Check sheet for the modelled part. Datum: model origin and axes. Units: mm. A direction names the side the tool comes from. Round coordinates to 2 decimals unless told otherwise and drop trailing zeros. Write each loop counter-clockwise with the first axis right and the second up, starting at its lowest first coordinate (ties: lowest second). Pieces come first, ordered by that corner, then holes. Notation, with made-up numbers: M 45.25,24.25 L 85.25,24.25 A22 cw 85.25,32.25 Z; hole C -24,4 d6. An arc over 180 degrees is marked long. One line per item, written item: value.
from build123d import *

# Parameters (mm, degrees)
F0_R     = 37
F0_R_2   = 35.5
F1_DEPTH = 1.5
F0_R_3   = 1.5
F2_DEPTH = 4


with BuildPart() as f1:
    # F0 (on Right) → F1 (new body, symmetric)
    with BuildSketch(Plane.YZ):
        Circle(F0_R)
        Circle(F0_R_2, mode=Mode.SUBTRACT)
    extrude(amount=F1_DEPTH, both=True)

    # F0 (on Right) → F2 (join, symmetric)
    with BuildSketch(Plane.YZ):
        Circle(F0_R_2)
        Circle(F0_R_3, mode=Mode.SUBTRACT)
    extrude(amount=F2_DEPTH, both=True)


solid = f1.part
Q1. Sectioned sample at D-D on z = 20. Enter the section's corners in (x, y).
Completed:
outline: M -4,-29.33 L -1.5,-29.33 L -1.5,-31.13 L 1.5,-31.13 L 1.5,-29.33 L 4,-29.33 L 4,29.33 L 1.5,29.33 L 1.5,31.13 L -1.5,31.13 L -1.5,29.33 L -4,29.33 Z
Q2. Sectioned sample at C-C on x = 3. Enter the section's corners in (y, z).
Completed:
outline: C 0,0 d71; hole C 0,0 d3
Q3. Sectioned sample at A-A on y = 0. Enter the section's corners in (x, z), and give its area (3 significant figures).
Completed:
outline: M -4,-35.5 L -1.5,-35.5 L -1.5,-37 L 1.5,-37 L 1.5,-35.5 L 4,-35.5 L 4,-1.5 L -4,-1.5 Z; M -4,1.5 L 4,1.5 L 4,35.5 L 1.5,35.5 L 1.5,37 L -1.5,37 L -1.5,35.5 L -4,35.5 Z
area: 553 mm^2
Q4. Depth check by flat-ended pin: P1, Ø1.8, axis at y = 0, z = 0, coming from the +X side; P2, Ø1, axis at x = 2.5, z = -26, coming from the -Y side; P3, Ø1.5, axis at x = 3, y = 14, coming from the -Z side; P4, Ø4, axis at x = 0, z = 7, coming from the -Y side. Enter the tip coordinate at first touch or a pass-through.
Completed:
P1: through
P2: y = -24.7
P3: z = -32.93
P4: y = -36.66
Q5. Scan lines: line 1 (Z direction, x = -1.25, y = 0); line 2 (Z direction, x = -2, y = -24); line 3 (Y direction, x = 0.75, z = 15.5). Record each from-to range of solid material in increasing order. Write a range as [from, to].
Completed:
line 1: [-37, -1.5], [1.5, 37]
line 2: [-26.16, 26.16]
line 3: [-33.6, 33.6]
Q6. Draft check along Y on faces 4 (the cylindrical face through (-2.732, -7.696, -34.656)), 5 (the cylindrical face through (-0.06, -1.5, 0.07)), 6 (the flat face through (-4, 0, -7)). Enter one of: pulls with the +Y half, pulls with the -Y half, needs draft (parallel to the pull), parting line crosses it, or undercut.
Completed:
face 4: parting line crosses it
face 5: undercut
face 6: needs draft
Q7. Access from +Z, -Z, +X, -X, +Y, -Y to the whole of each face (thin tool, end or side, straight path). Record for faces 1 (the cylindrical face through (2.768, -7.696, -34.656)), 2 (the flat face through (-1.5, -33, 14)), 3 (the flat face through (4, 0, -7)).
Completed:
face 1: +X
face 2: -X
face 3: +Z, -Z, +X, +Y, -Y
